Could you check a few things on this model? Use its own coordinates, in mm. A direction names the side the tool comes from. Coordinates: 2 decimals unless noted, no trailing zeros. Order: outer loops, then holes, each group sorted by start corner. A loop starts at its lowest first (then second) coordinate and runs counter-clockwise, first axis right, second up. Notation, with made-up numbers: (72.5, 69) -> (99.5, 69) arc R31 cw to (99.5, 104) -> close; hole circle Ø1 at (53, 8.25). An arc over 180 degrees is marked (long way). Use a Markdown table: item, result. Add a question column.
1) If we section it at D-D (z = 10): Write out the boundary of the cut face in (x, y).
2) If we section it at A-A (y = 38.1): Write out the boundary of the cut face in (x, z), plus the area to 3 significant figures.
3) Thinking about a two-plate mould opening in Y: for faces 1 (the flat face through (-1, -50.8, 1)), 2 (the flat face through (63.5, 0, 15)), 3 (the cylindrical face through (60.2, -38, 1.5)), which applies, +Y half, -Y half, draft (parallel to the pull), parting line (faces both ways), or undercut?
4) If we section it at C-C (y = 6): Write out the boundary of the cut face in (x, z), plus the area to 3 significant figures.
5) If I drill on L1, parallel to X at y = 38, z = 0.75; L2, parallel to Y at x = 63.5, z = 1.2; L3, parallel to Z at x = -12.5, y = -31.5, over which ranges is the centre line in solid material (lowest first)? Write a range as [from, to].
6) Which directions (+Z, -Z, +X, -X, +Y, -Y) give clear straight access to the entire face, cutting with the end or side of a thin tool? Please do faces 4 (the cylindrical face through (20.56, 18.24, 14.52)), 5 (the flat face through (-63.5, 0, 15)), 6 (the flat face through (-1, 31.75, 15)).
7) Will these pins go through, and if not, where does the flat tip stop? pin 1 Ø2.5 at (x, z) = (4, 14) entering from +Y; pin 2 Ø7.5 at (x, y) = (-63.5, 38.1) entering from +Z; pin 3 Ø3 at (y, z) = (13, 13.5) entering from +X.
8) If we section it at B-B (x = -39.5): Write out the boundary of the cut face in (y, z).
```python
from build123d import *

# Parameters (mm, degrees)
SKETCH1_W                      = 139.7
SKETCH1_H                      = 101.6
BOSS_EXTRUDE1_DEPTH            = 3
SKETCH2_R                      = 1
BOSS_EXTRUDE2_DEPTH            = 13
SKETCH3_W                      = 127
SKETCH3_H                      = 63.5
BOSS_EXTRUDE3_DEPTH            = 3
CUT_EXTRUDE1_DEPTH             = 88.342214879
CUT_EXTRUDE1_DEPTH_BACK        = 88.342214879
SKETCH4_R                      = 3.302
CUT_EXTRUDE2_REACH             = 89.839
SKETCH5_R                      = 2.2225
CUT_EXTRUDE2_DIRECTION_2_DEPTH = 88.838843913


with BuildPart() as part:
    # Sketch1 → Boss-Extrude1 (new body)
    with BuildSketch(Plane.XY):
        Rectangle(SKETCH1_W, SKETCH1_H)
    extrude(amount=BOSS_EXTRUDE1_DEPTH)

    # Sketch2 → Boss-Extrude2 (add)
    with BuildSketch(Plane.XY.offset(3)):
        with Locations(Location((-31.75, 25.4, 0), (0, 0, 180))):
            Circle(SKETCH2_R)
        with Locations(Location((31.75, 25.4, 0), (0, 0, 180))):
            Circle(SKETCH2_R)
        with Locations(Location((31.75, -25.4, 0), (0, 0, 180))):
            Circle(SKETCH2_R)
        with Locations(Location((-31.75, -25.4, 0), (0, 0, 180))):
            Circle(SKETCH2_R)
    extrude(amount=BOSS_EXTRUDE2_DEPTH)

    # Sketch3 → Boss-Extrude3 (add)
    with BuildSketch(Plane.XY.offset(16)):
        Rectangle(SKETCH3_W, SKETCH3_H)
    extrude(amount=-BOSS_EXTRUDE3_DEPTH)

    # Sketch4 → Cut-Extrude1 (cut, two sides: drawn at the far end of the back side and taken through both)
    with BuildSketch(Plane.XY.offset(3).offset(-CUT_EXTRUDE1_DEPTH_BACK)):
        with Locations((-63.5, -38.1)):
            Circle(SKETCH4_R)
        with Locations((63.5, 38.1)):
            Circle(SKETCH4_R)
        with Locations((-63.5, 38.1)):
            Circle(SKETCH4_R)
        with Locations((63.5, -38.1)):
            Circle(SKETCH4_R)
    extrude(amount=CUT_EXTRUDE1_DEPTH + CUT_EXTRUDE1_DEPTH_BACK, mode=Mode.SUBTRACT)

    # Sketch5 → Cut-Extrude2 (cut, up to next)
    with BuildSketch(Plane.XY.offset(16), mode=Mode.PRIVATE) as cut_extrude2_sk1:
        with Locations(Location((-59.5, 0, 0), (0, 0, 180))):
            Circle(SKETCH5_R)
    cut_extrude2_tool1 = extrude(cut_extrude2_sk1.sketch, amount=-CUT_EXTRUDE2_REACH, mode=Mode.PRIVATE) & part.part
    # Sketch5 → Cut-Extrude2 (cut, up to next)
    with BuildSketch(Plane.XY.offset(16), mode=Mode.PRIVATE) as cut_extrude2_sk2:
        with Locations(Location((18.338183986, -18.338183986, 0), (0, 0, 180))):
            Circle(SKETCH5_R)
    cut_extrude2_tool2 = extrude(cut_extrude2_sk2.sketch, amount=-CUT_EXTRUDE2_REACH, mode=Mode.PRIVATE) & part.part
    # Sketch5 → Cut-Extrude2 (cut, up to next)
    with BuildSketch(Plane.XY.offset(16), mode=Mode.PRIVATE) as cut_extrude2_sk3:
        with Locations(Location((18.338183986, 18.338183986, 0), (0, 0, 180))):
            Circle(SKETCH5_R)
    cut_extrude2_tool3 = extrude(cut_extrude2_sk3.sketch, amount=-CUT_EXTRUDE2_REACH, mode=Mode.PRIVATE) & part.part
    add(cut_extrude2_tool1.solids().sort_by_distance((-59.5, 0, 16))[0], mode=Mode.SUBTRACT)
    add(cut_extrude2_tool2.solids().sort_by_distance((18.338184, -18.338184, 16))[0], mode=Mode.SUBTRACT)
    add(cut_extrude2_tool3.solids().sort_by_distance((18.338184, 18.338184, 16))[0], mode=Mode.SUBTRACT)

    # Sketch5 → Cut-Extrude2 direction 2 (cut)
    with BuildSketch(Plane.XY.offset(16)):
        with Locations(Location((-59.5, 0, 0), (0, 0, 180))):
            Circle(SKETCH5_R)
        with Locations(Location((18.338183986, -18.338183986, 0), (0, 0, 180))):
            Circle(SKETCH5_R)
        with Locations(Location((18.338183986, 18.338183986, 0), (0, 0, 180))):
            Circle(SKETCH5_R)
    extrude(amount=CUT_EXTRUDE2_DIRECTION_2_DEPTH, mode=Mode.SUBTRACT)


solid = part.part
```
Answer sheet:
| question | item | result |
|---|---|---|
| 1 | outline | circle Ø2 at (-31.75, -25.4); circle Ø2 at (-31.75, 25.4); circle Ø2 at (31.75, -25.4); circle Ø2 at (31.75, 25.4) |
| 2 | outline | (-69.85, 0) -> (-66.8, 0) -> (-66.8, 3) -> (-69.85, 3) -> close; (-60.2, 0) -> (60.2, 0) -> (60.2, 3) -> (-60.2, 3) -> close; (66.8, 0) -> (69.85, 0) -> (69.85, 3) -> (66.8, 3) -> close |
| 2 | area | 379 mm2 |
| 3 | face 1 | -Y half |
| 3 | face 2 | draft |
| 3 | face 3 | undercut |
| 4 | outline | (-69.85, 0) -> (69.85, 0) -> (69.85, 3) -> (-69.85, 3) -> close; (-63.5, 13) -> (63.5, 13) -> (63.5, 16) -> (-63.5, 16) -> close |
| 4 | area | 800 mm2 |
| 5 | L1 | [-69.85, -66.8], [-60.2, 60.2], [66.8, 69.85] |
| 5 | L2 | [-50.8, -41.4], [-34.8, 34.8], [41.4, 50.8] |
| 5 | L3 | [0, 3], [13, 16] |
| 6 | face 4 | +Z |
| 6 | face 5 | +Z, -X, +Y, -Y |
| 6 | face 6 | +Z, +X, -X, +Y |
| 7 | pin 1 | y = 31.75 |
| 7 | pin 2 | z = 3 |
| 7 | pin 3 | x = 63.5 |
| 8 | outline | (-50.8, 0) -> (50.8, 0) -> (50.8, 3) -> (-50.8, 3) -> close; (-31.75, 13) -> (31.75, 13) -> (31.75, 16) -> (-31.75, 16) -> close |
